The model under review builds one solid part; all positions refer to its coordinate system, in mm. A direction names the side the tool comes from. Coordinates: 2 decimals unless noted, no trailing zeros. Order: outer loops, then holes, each group sorted by start corner. A loop starts at its lowest first (then second) coordinate and runs counter-clockwise, first axis right, second up. Notation, with made-up numbers: M 44.25,89 L 66.25,89 A11 cw 66.25,110 Z; hole C 9.25,-9.5 d7. An arc over 180 degrees is marked long. Answer in a Markdown table with one row per item.
from build123d import *

# Parameters (mm, degrees)
ESBO_O1_W                = 40
ESBO_O1_H                = 8
ESBO_O1_R                = 1.65
RESSALTO_EXTRUS_O1_DEPTH = 3
ESBO_O2_W                = 12
ESBO_O2_H                = 9
ESBO_O2_R                = 1.65
RESSALTO_EXTRUS_O2_DEPTH = 1.5
FILETE2_R                = 3
CORTE_EXTRUS_O1_REACH    = 25.854
ESBO_O3_R                = 2.6
ESPELHAR1_START          = 18.5
ESPELHAR1_OUTLINE_R      = 1.65
ESPELHAR1_DEPTH          = 1.5
ESPELHAR1_START_2        = 16.263932023
ESPELHAR1_2_OUTLINE_W    = 1
ESPELHAR1_2_OUTLINE_H    = 3
ESPELHAR1_2_DEPTH        = 2.236067977
ESPELHAR1_START_3        = -1
ESPELHAR1_3_DEPTH        = 4.84942
ESPELHAR1_START_4        = 3
ESPELHAR1_4_DEPTH        = 10


with BuildPart() as part:
    # Esboço1 → Ressalto-extrusão1 (new body)
    with BuildSketch(Plane.XY):
        Rectangle(ESBO_O1_W, ESBO_O1_H)
        with Locations((-16, 0)):
            Circle(ESBO_O1_R, mode=Mode.SUBTRACT)
        with Locations(Location((16, 0, 0), (0, 0, 180))):
            Circle(ESBO_O1_R, mode=Mode.SUBTRACT)
    extrude(amount=RESSALTO_EXTRUS_O1_DEPTH)

    # Esboço2 → Ressalto-extrusão2 (add)
    with BuildSketch(Plane.ZY.offset(20)):
        with Locations((6, -0.5)):
            Rectangle(ESBO_O2_W, ESBO_O2_H)
        with Locations((9, -1)):
            Circle(ESBO_O2_R, mode=Mode.SUBTRACT)
    extrude(amount=-RESSALTO_EXTRUS_O2_DEPTH)

    # Filete2
    # the kernel refuses this fillet: 3 mm, written as the material it adds along each edge
    with BuildSketch(Plane(origin=(-18.5, -4, 3), x_dir=(1, 0, 0), z_dir=(0, 0, -1))) as filete2_piece_1:
        with BuildLine():
            CenterArc((2.236067977, 3), FILETE2_R, 221.810314896, 48.189685104)
            Line((0, 1), (0, 0))
            Line((0, 0), (2.236067977, 0))
        make_face()
    extrude(amount=3)
    # the kernel refuses this fillet: 3 mm, written as the material it takes off along each edge
    with BuildSketch(Plane(origin=(-27.5, -5, 12), x_dir=(0, 0, -1), z_dir=(1, 0, 0))) as filete2_2_piece_1:
        with BuildLine():
            CenterArc((FILETE2_R, FILETE2_R), FILETE2_R, 180, 90)
            Line((0, FILETE2_R), (0, 0))
            Line((0, 0), (FILETE2_R, 0))
        make_face()
    extrude(amount=16.5, mode=Mode.SUBTRACT)
    with BuildSketch(Plane(origin=(-27.5, 4, 12), x_dir=(0, 0, -1), z_dir=(1, 0, 0))) as filete2_2_piece_2:
        with BuildLine():
            CenterArc((FILETE2_R, -FILETE2_R), FILETE2_R, 90, 90)
            Line((0, -FILETE2_R), (0, 0))
            Line((0, 0), (FILETE2_R, 0))
        make_face()
    extrude(amount=16.5, mode=Mode.SUBTRACT)

    # Corte-extrusão1: up to this face of the body (flat: up to its plane)
    corte_extrus_o1_end = Plane(part.part.faces().sort_by_distance((0.749892581, -0.010110038, 3))[0])
    # Esboço3 → Corte-extrusão1 (cut, up to the picked face)
    with BuildSketch(Plane.XY.offset(12), mode=Mode.PRIVATE) as corte_extrus_o1_sk1:
        with Locations((-16, 0)):
            Circle(ESBO_O3_R)
    corte_extrus_o1_tool1 = split(extrude(corte_extrus_o1_sk1.sketch, amount=-CORTE_EXTRUS_O1_REACH, mode=Mode.PRIVATE), bisect_by=corte_extrus_o1_end, keep=Keep.BOTH, mode=Mode.PRIVATE)
    add(corte_extrus_o1_tool1.solids().sort_by(Axis((-16, 0, 12), (0, 0, -1)))[0], mode=Mode.SUBTRACT)

    # Espelhar1: read off the stored shape, not the designer's step
    # Espelhar1 outline → Espelhar1 (add)
    with BuildSketch(Plane.YZ.offset(ESPELHAR1_START)):
        with BuildLine():
            Line((1, 12), (-2, 12))
            ThreePointArc((-2, 12), (-4.121320344, 11.121320344), (-5, 9))
            Line((-5, 9), (-5, 0))
            Line((-5, 0), (-4, 0))
            Line((-4, 0), (-4, 3))
            Line((-4, 3), (4, 3))
            Line((4, 3), (4, 9))
            ThreePointArc((4, 9), (3.121320344, 11.121320344), (1, 12))
        make_face()
        with Locations((-1, 9)):
            Circle(ESPELHAR1_OUTLINE_R, mode=Mode.SUBTRACT)
    extrude(amount=ESPELHAR1_DEPTH)

    # Espelhar1 2 outline → Espelhar1 2 (add)
    with BuildSketch(Plane.YZ.offset(ESPELHAR1_START_2)):
        with Locations((-4.5, 1.5)):
            Rectangle(ESPELHAR1_2_OUTLINE_W, ESPELHAR1_2_OUTLINE_H)
    extrude(amount=ESPELHAR1_2_DEPTH)

    # Espelhar1 3 outline → Espelhar1 3 (cut)
    with BuildSketch(Plane.XY.offset(ESPELHAR1_START_3)):
        with BuildLine():
            Line((16.263932023, -5), (18.5, -5))
            ThreePointArc((18.5, -5), (17.488676894, -4.261387212), (16.263932023, -4))
            Line((16.263932023, -4), (16.263932023, -5))
        make_face()
    extrude(amount=ESPELHAR1_3_DEPTH, mode=Mode.SUBTRACT)

    # Espelhar1 4 outline → Espelhar1 4 (cut)
    with BuildSketch(Plane.XY.offset(ESPELHAR1_START_4)):
        with BuildLine():
            Line((18.5, 0.714142843), (18.5, -0.714142843))
            ThreePointArc((18.5, -0.714142843), (18.6, 0), (18.5, 0.714142843))
        make_face()
    extrude(amount=ESPELHAR1_4_DEPTH, mode=Mode.SUBTRACT)


solid = part.part
(1) Take a section at C-C (y = 0). Write out the cut boundary in (x, z), then the cut area to 3 significant figures.
Report:
| item | result |
|---|---|
| outline | M -20,0 L -17.65,0 L -17.65,3 L -18.6,3 L -18.6,7.69 L -20,7.69 Z; M -20,10.31 L -18.6,10.31 L -18.6,12 L -20,12 Z; M -14.35,0 L 14.35,0 L 14.35,3 L -14.35,3 Z; M 17.65,0 L 20,0 L 20,7.69 L 18.6,7.69 L 18.6,3 L 17.65,3 Z; M 18.6,10.31 L 20,10.31 L 20,12 L 18.6,12 Z |
| area | 118 mm^2 |
(2) The part is to be moulded in two halves that separate along Y. For faces 1 (the cylindrical face through (-14.476, -0.632, 1.479)), 2 (the cylindrical face through (19.24, 3.14, 11.1)), 3 (the cylindrical face through (-17.505, -4.269, 1.521)), say which applies: +Y half, -Y half, draft (parallel to the pull), parting line (faces both ways), or undercut.
Report:
| item | result |
|---|---|
| face 1 | undercut |
| face 2 | +Y half |
| face 3 | -Y half |
(3) Take a section at A-A (z = 1.75). Write out the cut boundary in (x, y).
Report:
| item | result |
|---|---|
| outline | M -20,-5 L -18.5,-5 A3 cw -16.26,-4 L 16.26,-4 A3 cw 18.5,-5 L 20,-5 L 20,4 L -20,4 Z; hole C -16,0 d3.3; hole C 16,0 d3.3 |
(4) Insertion check: P1, Ø3, axis at y = -1, z = 9, coming from the -X side; P2, Ø4.5, axis at x = 2, y = -0.5, coming from the +Z side; P3, Ø2.5, axis at x = -1, z = 2, coming from the -Y side. Each pin has a flat end and moves straight along its axis. Give the tip position at first contact, or say it passes through.
Report:
| item | result |
|---|---|
| P1 | through |
| P2 | z = 3 |
| P3 | y = -4 |
(5) Take a section at B-B (z = 6.75). Write out the cut boundary in (x, y).
Report:
| item | result |
|---|---|
| outline | M -20,-5 L -18.5,-5 L -18.5,-0.71 A2.6 cw -18.5,0.71 L -18.5,4 L -20,4 Z; M 18.5,-5 L 20,-5 L 20,4 L 18.5,4 L 18.5,0.71 A2.6 cw 18.5,-0.71 Z |
(6) To check wall thickness, follow line 1 (Y direction, x = 19.4, z = 9); line 2 (X direction, y = 0.25, z = 2); line 3 (X direction, y = -1.25, z = 6.75). State the ranges of each line that lie inside material, in increasing order. Write a range as [from, to].
Report:
| item | result |
|---|---|
| line 1 | [-5, -2.65], [0.65, 4] |
| line 2 | [-20, -17.63], [-14.37, 14.37], [17.63, 20] |
| line 3 | [-20, -18.5], [18.5, 20] |
(7) Machinability: for faces 4 (the flat face through (0, -1, 0)), 5 (the flat face through (0, -4, 1)), 6 (the cylindrical face through (-19.26, -4.1, 11.14)), 7 (the cylindrical face through (18.6, 0, 6.4)), 8 (the flat face through (-18.5, -3, 6)), which of the approach directions +Z, -Z, +X, -X, +Y, -Y give a long, thin tool a straight path to every point of the face, cutting with its end or side? Answer none if there is none.
Report:
| item | result |
|---|---|
| face 4 | -Z, +X, -X, +Y, -Y |
| face 5 | +Z, -Z, -Y |
| face 6 | +Z, +X, -X, -Y |
| face 7 | +Z |
| face 8 | +Z, +Y, -Y |
(8) Take a section at D-D (z = 10). Write out the cut boundary in (x, y), then the cut area to 3 significant figures.
Report:
| item | result |
|---|---|
| outline | M -20,-4.83 L -18.5,-4.83 L -18.5,-2.31 L -20,-2.31 Z; M -20,0.31 L -18.58,0.31 A2.6 cw -18.5,0.71 L -18.5,3.83 L -20,3.83 Z; M 18.5,-4.83 L 20,-4.83 L 20,-2.31 L 18.5,-2.31 Z; M 18.5,0.71 A2.6 cw 18.58,0.31 L 20,0.31 L 20,3.83 L 18.5,3.83 Z |
| area | 18.1 mm^2 |
